Input: dimensioned drawing with shaded views. Units: mm. Origin: part minimum x, y, z. Give positions to 0.01 mm unless a question says otherwise; leave off trailing zeros. Loops run counter-clockwise (first coordinate to the right, second up) from the corner with the lowest first, then second, coordinate; pieces in that order, holes last. Notation, with made-up numbers: (49.5, -19.5) -> (87.5, -19.5) arc R23 ccw to (87.5, 14.5) -> close; hole circle Ø11 at (73, 0.25). An arc over 180 degrees is marked (long way). Answer as a JSON object with one key per item and string values.
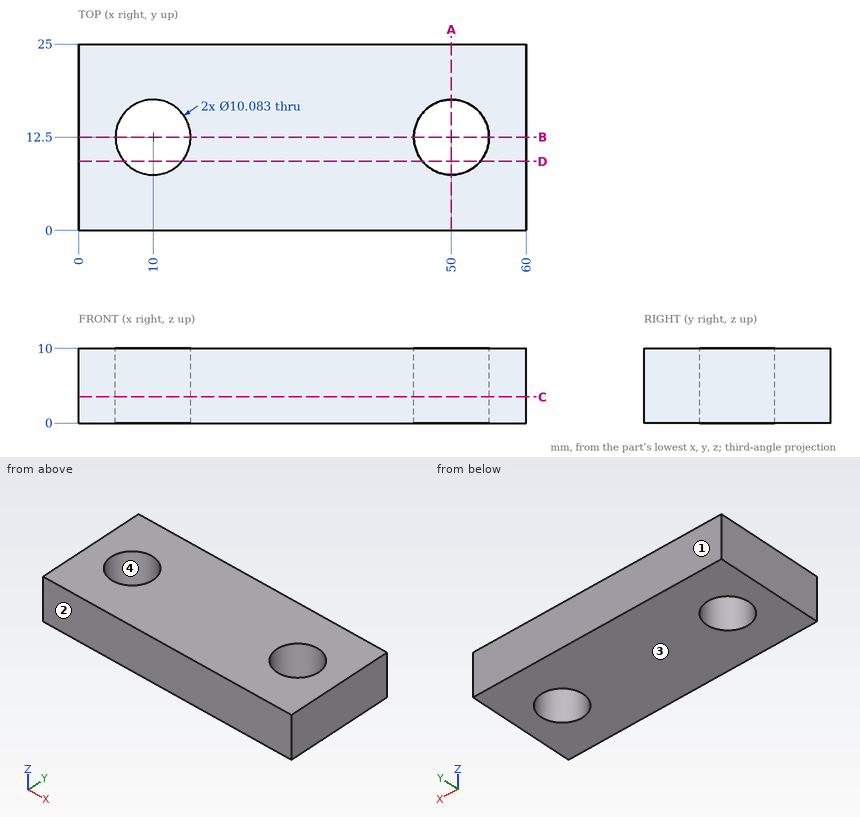
Q1. Section C-C, the plane z = 3.5. Return the cut outline in (x, y), then the cut area to 3 significant figures.
Evaluation:
{"outline": "(0, 0) -> (60, 0) -> (60, 25) -> (0, 25) -> close; hole circle Ø10.08 at (10, 12.5); hole circle Ø10.08 at (50, 12.5)", "area": "1,340 mm2"}
Q2. Section A-A, the plane x = 50. Return the cut outline in (y, z).
Evaluation:
{"outline": "(0, 0) -> (7.46, 0) -> (7.46, 10) -> (0, 10) -> close; (17.54, 0) -> (25, 0) -> (25, 10) -> (17.54, 10) -> close"}
Q3. Ray query, line 1 along X through (y, z) = (12.5, 2.75); line 2 along X through (y, z) = (9.5, 1); line 3 along Y through (x, z) = (50, 8). Return the intervals inside material, ascending.
Evaluation:
{"line 1": "x = 0 to 4.96, 15.04 to 44.96, 55.04 to 60", "line 2": "x = 0 to 5.95, 14.05 to 45.95, 54.05 to 60", "line 3": "y = 0 to 7.46, 17.54 to 25"}
Q4. Draft query along Y for the marked faces 1, 2, 3 and 4. Return one class per face: +Y half, -Y half, draft (parallel to the pull), parting line (faces both ways), or undercut.
Evaluation:
{"face 1": "+Y half", "face 2": "-Y half", "face 3": "draft", "face 4": "undercut"}
Q5. Section D-D, the plane y = 9.25. Return the cut outline in (x, z).
Evaluation:
{"outline": "(0, 0) -> (6.15, 0) -> (6.15, 10) -> (0, 10) -> close; (13.85, 0) -> (46.15, 0) -> (46.15, 10) -> (13.85, 10) -> close; (53.85, 0) -> (60, 0) -> (60, 10) -> (53.85, 10) -> close"}
Q6. Section B-B, the plane y = 12.5. Return the cut outline in (x, z).
Evaluation:
{"outline": "(0, 0) -> (4.96, 0) -> (4.96, 10) -> (0, 10) -> close; (15.04, 0) -> (44.96, 0) -> (44.96, 10) -> (15.04, 10) -> close; (55.04, 0) -> (60, 0) -> (60, 10) -> (55.04, 10) -> close"}
